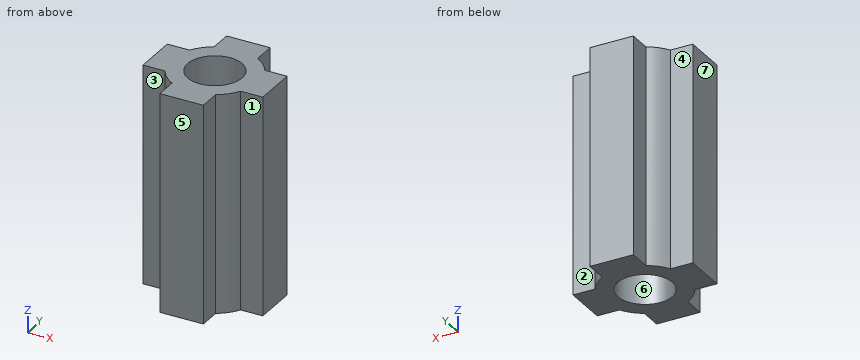
Autodesk Inventor part; units mm, degrees
ref_plane "Plano de trabajo1" through (0, 0, 11) normal (0, 0, 1) x (1, 0, 0)
ref_plane "YZ Plane" through (0, 0, 0) normal (1, 0, 0) x (0, 1, 0)
ref_plane "XZ Plane" through (0, 0, 0) normal (0, 1, 0) x (-1, 0, 0)
sketch "Boceto3" plane through (0, 0, 0) normal (0, 0, 1) x (1, 0, 0)
  circle A0 centre (0, 0) radius 2
  dimension "d13" = 4
sketch "Boceto1" plane through (0, 0, 0) normal (0, 0, 1) x (1, 0, 0)
  line L0 (-1, 2.7591) -> (1, 2.7591)
  line L1 (1, 2.7591) -> (1, -2.7409)
  line L2 (1, -2.7409) -> (-1, -2.7409)
  line L3 (-1, -2.7409) -> (-1, 2.7591)
  line L4 (0, 5.941) -> (0, -7.9228)
  line L5 (-6.4273, 0.0091) -> (13.1091, 0.0091)
  line L6 (-2.75, 1.0091) -> (2.75, 1.0091)
  line L7 (2.75, 1.0091) -> (2.75, -0.9909)
  line L8 (2.75, -0.9909) -> (-2.75, -0.9909)
  line L9 (-2.75, -0.9909) -> (-2.75, 1.0091)
  point P0 (0, 0)
  point P1 (0, 2.7591)
  point P2 (1, 0.0091)
  point P3 (-2.75, 0.0091)
  point P4 (0, -0.9909)
  dimension "d0" = 2
  dimension "d1" = 5.5
  dimension "d2" = 5.5
  dimension "d3" = 2
ref_plane "Plano de trabajo1" through (0, 0, 11) normal (0, 0, 1) x (1, 0, 0)
extrude "Extrusión2" add sketch "Boceto1" along normal blind 10
extrude "Extrusión3" add sketch "Boceto3" along normal blind 10
sketch "Boceto2" plane through (0, 0, 10) normal (0, 0, 1) x (1, 0, 0)
  point P0 (0, 0)
  point P1 (0, 0)
hole "Agujero1" at (0, 0, 10) direction (0, 0, -1) diameter 2.5 end through all
properties part number "motor_axis_cross_2.5" material "Plástico ABS"
The model under review builds one solid part; all positions refer to its coordinate system, in mm. Face numbers are marked on the shaded views. A direction names the side the tool comes from. Give positions to 0.01 mm unless a question says otherwise; leave off trailing zeros. Write each loop counter-clockwise with the first axis right and the second up, starting at its lowest first coordinate (ties: lowest second). Pieces come first, ordered by that corner, then holes. Notation, with made-up numbers: (68.5, 9) - (90.5, 9) arc R22 ccw to (90.5, 46) - close; hole circle Ø6 at (-38, 19). An arc over 180 degrees is marked (long way). Answer in a Markdown table with one row per item. Add a question column.
1. Insertion check: P1, Ø0.8, axis at x = -2, z = 5.5, coming from the +Y side; P2, Ø1.1, axis at y = 2, z = 5, coming from the +X side; P3, Ø0.8, axis at y = -2, z = 5, coming from the -X side. Each pin has a flat end and moves straight along its axis. Give the tip position at first contact, or say it passes through.
2. We need section C-C on y = 0. Write out the cut boundary in (x, z).
3. We need section A-A on x = 0.35. Write out the cut boundary in (y, z).
4. Tool access review of the marked faces 1, 2, 3 and 4: name each direction out of +Z, -Z, +X, -X, +Y, -Y from which nothing blocks a thin tool from reaching the whole face with its end or side.
5. Draft analysis for pull direction X (two halves, no side actions). For the marked faces 5, 6 and 7, state which applies: +X half, -X half, draft (parallel to the pull), parting line (faces both ways), or undercut.
6. Wall thickness on line 1 along Y through (x, z) = (0, 4.75); line 2 along X through (y, z) = (0, 6.75); line 3 along X through (y, z) = (2.5, 7): over which ranges is each line inside the solid? List them lowest first. Write a range as [from, to].
7. We need section D-D on x = 1.9. Write out the cut boundary in (y, z).
8. We need section B-B on z = 2. Write out the cut boundary in (x, y), then the cut area to 3 significant figures.
Ans:
| question | item | result |
|---|---|---|
| 1 | P1 | stops at y = 1.2 |
| 1 | P2 | stops at x = 1.38 |
| 1 | P3 | stops at x = -1.2 |
| 2 | outline | (-2.75, 0) - (-1.25, 0) - (-1.25, 10) - (-2.75, 10) - close; (1.25, 0) - (2.75, 0) - (2.75, 10) - (1.25, 10) - close |
| 3 | outline | (-2.74, 0) - (-1.2, 0) - (-1.2, 10) - (-2.74, 10) - close; (1.2, 0) - (2.76, 0) - (2.76, 10) - (1.2, 10) - close |
| 4 | face 1 | +Z, -Z, +X, -Y |
| 4 | face 2 | +Z, -Z, +X, +Y |
| 4 | face 3 | +Z, -Z, -X, -Y |
| 4 | face 4 | +Z, -Z, -X, +Y |
| 5 | face 5 | draft |
| 5 | face 6 | undercut |
| 5 | face 7 | -X half |
| 6 | line 1 | y = [-2.74, -1.25], [1.25, 2.76] |
| 6 | line 2 | x = [-2.75, -1.25], [1.25, 2.75] |
| 6 | line 3 | x = [-1, 1] |
| 7 | outline | (-0.99, 0) - (1.01, 0) - (1.01, 10) - (-0.99, 10) - close |
| 8 | outline | (-2.75, -0.99) - (-1.74, -0.99) arc R2 ccw to (-1, -1.73) - (-1, -2.74) - (1, -2.74) - (1, -1.73) arc R2 ccw to (1.74, -0.99) - (2.75, -0.99) - (2.75, 1.01) - (1.73, 1.01) arc R2 ccw to (1, 1.73) - (1, 2.76) - (-1, 2.76) - (-1, 1.73) arc R2 ccw to (-1.73, 1.01) - (-2.75, 1.01) - close; hole circle Ø2.5 at (0, 0) |
| 8 | area | 14.4 mm^2 |
